```python
from build123d import *

# Parameters (mm, degrees)
SKETCH1_W           = 200
SKETCH1_H           = 150
BOSS_EXTRUDE1_DEPTH = 1
SKETCH2_R           = 1.5
SKETCH2_R_2         = 1.4
SKETCH2_W           = 14
SKETCH2_H           = 7
SKETCH2_W_2         = 12
SKETCH2_H_2         = 3
SKETCH2_W_3         = 23
SKETCH2_H_3         = 13.5
CUT_EXTRUDE1_DEPTH  = 1


with BuildPart() as part:
    # Sketch1 → Boss-Extrude1 (new body)
    with BuildSketch(Plane.XY):
        Rectangle(SKETCH1_W, SKETCH1_H)
    extrude(amount=BOSS_EXTRUDE1_DEPTH)

    # Sketch2 → Cut-Extrude1 (cut)
    with BuildSketch(Plane.XY.offset(1)):
        with Locations((-76.53, -67.5)):
            Circle(SKETCH2_R)
        with Locations((-59.53, -67.5)):
            Circle(SKETCH2_R)
        with Locations(Location((-59.53, 67.5, 0), (0, 0, 180))):
            Circle(SKETCH2_R)
        with Locations(Location((-76.53, 67.5, 0), (0, 0, 180))):
            Circle(SKETCH2_R)
        with Locations((-73, -40)):
            Circle(SKETCH2_R)
        with Locations((-63, -40)):
            Circle(SKETCH2_R)
        with Locations((-88.25346752, -58)):
            Circle(SKETCH2_R)
        with Locations((66.74653248, -58)):
            Circle(SKETCH2_R)
        with Locations(Location((66.74653248, 58, 0), (0, 0, 180))):
            Circle(SKETCH2_R)
        with Locations(Location((-88.25346752, 58, 0), (0, 0, 180))):
            Circle(SKETCH2_R)
        with Locations((64.8, 68.5)):
            Circle(SKETCH2_R_2)
        with Locations((92.2, 68.5)):
            Circle(SKETCH2_R_2)
        with Locations((-68, -55.5)):
            Rectangle(SKETCH2_W, SKETCH2_H)
        with Locations((-68, 55.5)):
            Rectangle(SKETCH2_W, SKETCH2_H)
        with Locations((-27, -13.75)):
            Rectangle(SKETCH2_W_2, SKETCH2_H_2)
        with Locations((-27, 13.75)):
            Rectangle(SKETCH2_W_2, SKETCH2_H_2)
        with Locations((78.5, 68.25)):
            Rectangle(SKETCH2_W_3, SKETCH2_H_3)
    extrude(amount=-CUT_EXTRUDE1_DEPTH, mode=Mode.SUBTRACT)


solid = part.part
```
Source: CAD feature listing. Evaluate the final solid. Frame: model axes, mm. Give positions to 0.01 mm unless a question says otherwise; leave off trailing zeros. Loops run counter-clockwise (first coordinate to the right, second up) from the corner with the lowest first, then second, coordinate; pieces in that order, holes last. Notation, with made-up numbers: (28, 9.25) -> (35, 9.25) arc R27 ccw to (35, 40.25) -> close; hole circle Ø4 at (14, -35). An arc over 180 degrees is marked (long way). Put each result on its own line as item: value. Start each with the question number.
1) Cut plane B-B (z = 0.2). State how many separate pieces and enclosed holes the cut face has, then the cut area to 3 significant figures.
2) Contact query for a flat-ended pin moving along its axis: P1, Ø1.8, axis at x = -73, y = -40, coming from the -Z side. Output: stop coordinate, or through.
3) Material intervals for probe 1 along Y at (x, z) = (-76.53, 0.75); probe 2 along Y at (x, z) = (-63, 0.3); probe 3 along X at (y, z) = (58, 0.2), sorted ascending.
4) Cut plane A-A (x = -30). Return loops of the section in (y, z).
Results are:
1. separate pieces: 1
1. enclosed holes: 16
1. area: 29,300 mm2
2. P1: passes through
3. probe 1: y = -75 to -69, -66 to 66, 69 to 75
3. probe 2: y = -75 to -59, -52 to -41.5, -38.5 to 52, 59 to 75
3. probe 3: x = -100 to -89.75, -86.75 to -75, -61 to 65.25, 68.25 to 100
4. outline: (-75, 0) -> (-15.25, 0) -> (-15.25, 1) -> (-75, 1) -> close; (-12.25, 0) -> (12.25, 0) -> (12.25, 1) -> (-12.25, 1) -> close; (15.25, 0) -> (75, 0) -> (75, 1) -> (15.25, 1) -> close
